Autodesk Fusion 360 part; units mm, degrees
sketch "스케치1" plane through (0, 0, 0) normal (0, 0, 1) x (1, 0, 0)
  line L0 (0, 0) -> (100, 0)
  line L1 (100, 0) -> (100, 100)
  line L2 (100, 100) -> (0, 100)
  line L3 (0, 100) -> (0, 0)
  dimension "d1" = 100
  dimension "d2" = 100
extrude "돌출1" add sketch "스케치1" along normal blind 2
sketch "스케치2" plane through (0, 0, 2) normal (0, 0, 1) x (-1, 0, 0)
  line L0 (0, -100) -> (-100, -100)
  line L1 (-100, -100) -> (-100, 0)
  line L2 (-100, 0) -> (0, 0)
  line L3 (0, 0) -> (0, -100)
  line L4 (-10, -98) -> (-90, -98)
  line L5 (-98, -90) -> (-98, -10)
  line L6 (-90, -2) -> (-10, -2)
  line L7 (-2, -10) -> (-2, -90)
  line L8 (-2, -90) -> (-10, -90)
  line L9 (-10, -90) -> (-10, -98)
  line L10 (-90, -98) -> (-90, -90)
  line L11 (-90, -90) -> (-98, -90)
  line L12 (-98, -10) -> (-90, -10)
  line L13 (-90, -10) -> (-90, -2)
  line L14 (-10, -2) -> (-10, -10)
  line L15 (-10, -10) -> (-2, -10)
  point P0 (0, -100)
  point P1 (-100, 0)
  dimension "d5" = 2
  dimension "d6" = 2
  dimension "d7" = 8
  dimension "d8" = 8
  dimension "d9" = 2
  dimension "d10" = 2
  dimension "d11" = 8
  dimension "d12" = 8
extrude "돌출2" add sketch "스케치2" along normal blind 8
sketch "스케치3" plane through (0, 0, 10) normal (0, 0, 1) x (-1, 0, 0)
  circle A0 centre (-5, -95) radius 1.5
  circle A1 centre (-95, -95) radius 1.5
  circle A2 centre (-95, -5) radius 1.5
  circle A3 centre (-5, -5) radius 1.5
  dimension "d15" = 3
  dimension "d16" = 5
  dimension "d17" = 5
  dimension "d18" = 90
  dimension "d19" = 90
extrude "돌출3" cut sketch "스케치3" against normal blind 10
fillet "필렛1" radius 3 4 edges at (0, 0, 5) (100, 0, 5) (100, 100, 5) (0, 100, 5)
fillet "필렛1" radius 3 4 edges at (10, 90, 6) (10, 10, 6) (90, 90, 6) (90, 10, 6)
chamfer "챔퍼1" distance 2 angle 45 4 edges at (6.3985, 95.5424, 0) (6.3985, 5.5424, 0) (96.3985, 5.5424, 0) (96.3985, 95.5424, 0)
sketch "스케치4" plane through (0, 0, 2) normal (0, 0, 1) x (-1, 0, 0)
  line L0 (-39.5, -60.3) -> (-80.5, -60.3)
  line L1 (-80.5, -60.3) -> (-80.5, -39.7)
  line L2 (-80.5, -39.7) -> (-39.5, -39.7)
  line L3 (-39.5, -39.7) -> (-39.5, -60.3)
  circle A0 centre (-35.5, -55.1) radius 2.25
  circle A1 centre (-35.5, -45.1) radius 2.25
  circle A2 centre (-84.5, -55.1) radius 2.25
  circle A3 centre (-84.5, -45.1) radius 2.25
  circle A4 centre (-25, -50) radius 5
  point P0 (-3, -100)
  dimension "d27" = 20.6
  dimension "d28" = 41
  dimension "d29" = 39.5
  dimension "d33" = 10
  dimension "d34" = 49
  dimension "d35" = 4.5
  dimension "d37" = 5.4
  dimension "d41" = 39.7
  dimension "d43" = 4
  dimension "d45" = 10
  dimension "d46" = 25
  dimension "d47" = 50
extrude "돌출4" cut sketch "스케치4" against normal blind 2
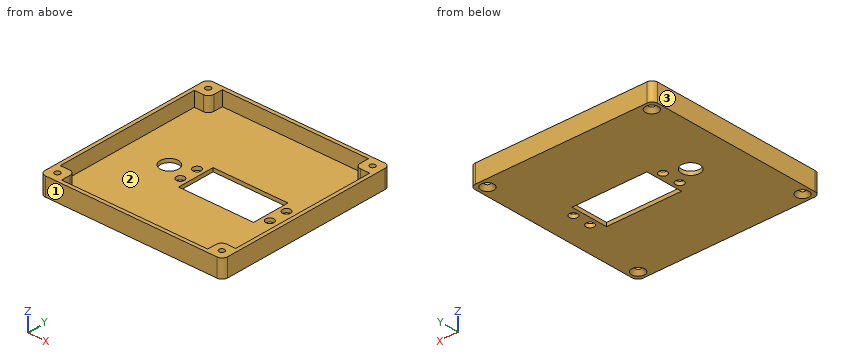
CAD build for the part. Positions are in the model's coordinates, mm. Face numbers are marked on the shaded views. Round coordinates to 2 decimals unless told otherwise and drop trailing zeros. Order: outer loops, then holes, each group sorted by start corner. A loop starts at its lowest first (then second) coordinate and runs counter-clockwise, first axis right, second up. Notation, with made-up numbers: (30, 43.25) -> (53, 43.25) arc R25 ccw to (53, 63.25) -> close; hole circle Ø6 at (-38.75, 64). An arc over 180 degrees is marked (long way). One line per question, with ' | ' between items.
Q1. Probe probe 1 along Y at (x, z) = (35.5, 0.75); probe 2 along X at (y, z) = (95, 8). List the from-to ranges inside material, lowest first.
Completed:
probe 1: y = 0 to 42.85, 47.35 to 52.85, 57.35 to 100 | probe 2: x = 0 to 3.5, 6.5 to 10, 90 to 93.5, 96.5 to 100
Q2. Slice it at C-C (z = 4). Write the cut outline in (x, y), then the cut area to 3 significant figures.
Completed:
outline: (0, 3) arc R3 ccw to (3, 0) -> (97, 0) arc R3 ccw to (100, 3) -> (100, 97) arc R3 ccw to (97, 100) -> (3, 100) arc R3 ccw to (0, 97) -> close; hole (2, 10) -> (7, 10) arc R3 cw to (10, 7) -> (10, 2) -> (90, 2) -> (90, 7) arc R3 cw to (93, 10) -> (98, 10) -> (98, 90) -> (93, 90) arc R3 cw to (90, 93) -> (90, 98) -> (10, 98) -> (10, 93) arc R3 cw to (7, 90) -> (2, 90) -> close; hole circle Ø3 at (5, 5); hole circle Ø3 at (5, 95); hole circle Ø3 at (95, 5); hole circle Ø3 at (95, 95) | area: 996 mm^2
Q3. Drop flat-ended pins along their axis: pin 1 (2.5 mm diameter, centred on y = 95.5, z = 6.5, fed in from -X); pin 2 (2.5 mm diameter, centred on x = 95, y = 95, fed in from +Z); pin 3 (5 mm diameter, centred on x = 18.5, y = 78.5, fed in from +Z). Give the stop position or say it passes through.
Completed:
pin 1: stops at x = 0 | pin 2: passes through | pin 3: stops at z = 2
Q4. Slice it at A-A (y = 95). Write the cut outline in (x, z).
Completed:
outline: (0, 0) -> (1.5, 0) -> (3.5, 2) -> (3.5, 10) -> (0, 10) -> close; (6.5, 2) -> (8.5, 0) -> (91.5, 0) -> (93.5, 2) -> (93.5, 10) -> (90, 10) -> (90, 2) -> (10, 2) -> (10, 10) -> (6.5, 10) -> close; (96.5, 2) -> (98.5, 0) -> (100, 0) -> (100, 10) -> (96.5, 10) -> close
Q5. Two-plate mould, pull along X, no slides. Class the marked faces 1, 2 and 3: released by +X, released by -X, zero draft, split by the parting line, or undercut.
Completed:
face 1: zero draft | face 2: undercut | face 3: released by -X
Q6. Slice it at B-B (x = 25). Write the cut outline in (y, z), then the cut area to 3 significant figures.
Completed:
outline: (0, 0) -> (45, 0) -> (45, 2) -> (2, 2) -> (2, 10) -> (0, 10) -> close; (55, 0) -> (100, 0) -> (100, 10) -> (98, 10) -> (98, 2) -> (55, 2) -> close | area: 212 mm^2
